Autodesk Inventor part; units mm, degrees
ref_plane "YZ Plane" through (0, 0, 0) normal (1, 0, 0) x (0, 1, 0)
ref_plane "XZ Plane" through (0, 0, 0) normal (0, 1, 0) x (-1, 0, 0)
ref_plane "XY Plane" through (0, 0, 0) normal (0, 0, 1) x (1, 0, 0)
sketch "Sketch1" plane through (0, 0, 0) normal (0, 0, 1) x (1, 0, 0)
  line L0 (-25.4, 45.4025) -> (-25.4, -24.4475)
  line L1 (-22.225, -27.6225) -> (22.225, -27.6225)
  line L2 (25.4, -24.4475) -> (25.4, 45.4025)
  line L3 (22.225, 48.5775) -> (-22.225, 48.5775)
  line L4 (0, 57.3133) -> (0, -29.6676)
  circle A0 centre (-12.5413, 35.8775) radius 2.54
  circle A1 centre (12.5412, 35.8775) radius 2.54
  arc A2 (-25.4, -24.4475) -> (-22.225, -27.6225) centre (-22.225, -24.4475) ccw
  arc A3 (22.225, -27.6225) -> (25.4, -24.4475) centre (22.225, -24.4475) ccw
  arc A4 (25.4, 45.4025) -> (22.225, 48.5775) centre (22.225, 45.4025) ccw
  arc A5 (-22.225, 48.5775) -> (-25.4, 45.4025) centre (-22.225, 45.4025) ccw
  line L5 (-55.0388, 0) -> (75.1356, 0)
  point P0 (-25.4, 48.5775)
  point P1 (-25.4, -27.6225)
  point P2 (25.4, -27.6225)
  point P3 (25.4, 48.5775)
  dimension "d10" = 50.8
  dimension "d11" = 76.2
  dimension "d12" = 5.08
  dimension "d13" = 25.0825
  dimension "d18" = 3.175
extrude "Extrusion2" add sketch "Sketch1" along normal blind 6.35
sketch "Sketch2" plane through (0, 0, 6.35) normal (0, 0, 1) x (1, 0, 0)
  line L0 (15.209, -21.209) -> (-15.209, -21.209)
  line L1 (-21.209, -15.209) -> (-21.209, 15.209)
  line L2 (-15.209, 21.209) -> (15.209, 21.209)
  line L3 (21.209, 15.209) -> (21.209, -15.209)
  line L4 (21.209, -21.209) -> (-21.209, 21.209) construction
  line L5 (-21.209, -21.209) -> (21.209, 21.209) construction
  line L6 (-21.209, 15.209) -> (-15.209, 21.209)
  line L7 (21.209, 15.209) -> (15.209, 21.209)
  line L8 (21.209, -15.209) -> (15.209, -21.209)
  line L9 (-15.209, -21.209) -> (-21.209, -15.209)
  point P0 (0, 0)
  dimension "d24" = 42.418
  dimension "d25" = 42.418
  dimension "d26" = 6
  dimension "d27" = 6
  dimension "d28" = 6
  dimension "d29" = 6
  dimension "d30" = 6
  dimension "d31" = 6
  dimension "d32" = 6
  dimension "d33" = 6
extrude "Extrusion3" cut sketch "Sketch2" against normal up to next
sketch "Sketch3" plane through (0, 0, 6.35) normal (0, 0, 1) x (1, 0, 0)
  line L0 (0, 74.5248) -> (0, -62.4529)
  line L1 (-21.209, 4.2436) -> (-23.241, 4.2436)
  line L2 (-23.241, 4.2436) -> (-23.241, -5.3802)
  line L3 (-23.241, -5.3802) -> (-21.209, -5.3802)
  line L4 (-21.209, -5.3802) -> (-21.209, 4.2436)
  line L5 (-21.209, 15.209) -> (-21.209, -15.209)
  line L6 (21.209, 4.2436) -> (23.241, 4.2436)
  line L7 (23.241, 4.2436) -> (23.241, -5.3802)
  line L8 (23.241, -5.3802) -> (21.209, -5.3802)
  line L9 (21.209, -5.3802) -> (21.209, 4.2436)
  point P0 (0, 0)
  point P1 (-21.209, 0)
  point P2 (21.209, 0)
  dimension "d39" = 2.032
extrude "Extrusion4" cut sketch "Sketch3" against normal up to next
fillet "Fillet1" radius 1.27 4 edges at (-23.241, 4.2436, 3.175) (-23.241, -5.3802, 3.175) (23.241, 4.2436, 3.175) (23.241, -5.3802, 3.175)
equation "\"d25\" = d24"
equation "\"d27\" = d26"
equation "\"d28\" = d26"
equation "\"d29\" = d28"
equation "\"d30\" = d26"
equation "\"d31\" = d30"
equation "\"d32\" = d26"
equation "\"d33\" = d32"
properties part number "Motor_Clamp"
Can you work these out from the model? Positions are in its coordinate system, mm. A direction names the side the tool comes from. Give positions to 0.01 mm unless a question says otherwise; leave off trailing zeros. Loops run counter-clockwise (first coordinate to the right, second up) from the corner with the lowest first, then second, coordinate; pieces in that order, holes last. Notation, with made-up numbers: M -2.5,48.25 L 12.5,48.25 A13 ccw 12.5,72.25 Z; hole C -21,2.25 d6. An arc over 180 degrees is marked long. One line per item, written item: value.
1) On a 3-axis mill with a long thin cutter (end or side, diameter ignored), from which of +Z, -Z, +X, -X, +Y, -Y can I reach the whole of each face in a straight line? I mean faces 4 (the face through (-18.25, 18.17, 3.22)), 5 (the face through (0, -27.622, 3)). Say none if no direction works.
Geometry check:
face 4: +Z, -Z
face 5: +Z, -Z, +X, -X, -Y
2) I'm going to push a flat-ended pin straight in: pin 1 (3 mm diameter, centred on x = -14, y = 32, fed in from -Z). Where does the tip first touch, or does it pass through?
Geometry check:
pin 1: stops at z = 0
3) Imagine slicing it at B-B on y = -1.5. Write out the boundary of the cut face in (x, z), and give its area (3 significant figures).
Geometry check:
outline: M -25.4,0 L -23.24,0 L -23.24,6.35 L -25.4,6.35 Z; M 23.24,0 L 25.4,0 L 25.4,6.35 L 23.24,6.35 Z
area: 27.4 mm²
4) Thinking about a two-plate mould opening in Y: for faces 1 (the face through (0, 21.209, 3)), 2 (the face through (-25.4, 11, 3)), 3 (the face through (24.49, -26.67, 3.13)), which applies, +Y half, -Y half, draft (parallel to the pull), parting line (faces both ways), or undercut?
Geometry check:
face 1: undercut
face 2: draft
face 3: -Y half
5) Imagine slicing it at C-C on z = 1.5. Count the separate pieces of the cut face and the enclosed holes in it, and give its area (3 significant figures).
Geometry check:
separate pieces: 1
enclosed holes: 3
area: 2,060 mm²
6) Please list where these lines run through material, in increasing order: line 1 (Y direction, x = -3, z = 2.5); line 2 (Y direction, x = -12.5, z = 1.75); line 3 (Y direction, x = 11.5, z = 2.75).
Geometry check:
line 1: y = -27.62 to -21.21, 21.21 to 48.58
line 2: y = -27.62 to -21.21, 21.21 to 33.34, 38.42 to 48.58
line 3: y = -27.62 to -21.21, 21.21 to 33.56, 38.19 to 48.58
7) Imagine slicing it at A-A on x = 1.5. Write out the boundary of the cut face in (y, z).
Geometry check:
outline: M -27.62,0 L -21.21,0 L -21.21,6.35 L -27.62,6.35 Z; M 21.21,0 L 48.58,0 L 48.58,6.35 L 21.21,6.35 Z
8) Imagine slicing it at D-D on x = 11. Write out the boundary of the cut face in (y, z).
Geometry check:
outline: M -27.62,0 L -21.21,0 L -21.21,6.35 L -27.62,6.35 Z; M 21.21,0 L 33.86,0 L 33.86,6.35 L 21.21,6.35 Z; M 37.9,0 L 48.58,0 L 48.58,6.35 L 37.9,6.35 Z
